Work out the finished part from the listing and answer in its coordinate system (mm). A direction names the side the tool comes from. Round coordinates to 2 decimals unless told otherwise and drop trailing zeros. Loops run counter-clockwise (first coordinate to the right, second up) from the corner with the lowest first, then second, coordinate; pieces in that order, holes last. Notation, with made-up numbers: (23.25, 66.5) -> (28.25, 66.5) arc R22 ccw to (28.25, 90.5) -> close; hole circle Ø2 at (-30, 17.25). An arc over 180 degrees is marked (long way). Write item = value, one per line. Start each with the question number.
```python
from build123d import *

# Parameters (mm, degrees)
F3_DEPTH = 12.13


with BuildPart() as f1:
    # F0 (on Front) → F1 (revolve)
    with BuildSketch(Plane.XZ):
        Polygon((20.5, 23.07), (20.5, 0), (23.37, 0), (23.37, 12.13), (21.62, 12.13), (21.62, 23.07), align=None)
    revolve(axis=Axis((0, 0, 6.4205313101), (0, 0, 1)))

    # F2 (on face) → F3 (join)
    with BuildSketch(Plane(origin=(0, 0, 0), x_dir=(1, 0, 0), z_dir=(0, 0, -1))):
        with BuildLine():
            ThreePointArc((-2.035, 23.2812301007), (0, 23.37), (2.035, 23.2812301007))
            ThreePointArc((2.035, 23.2812301007), (0, 25.37), (-2.035, 23.2812301007))
        make_face()
        with BuildLine():
            ThreePointArc((-7.9912848, 21.9612446652), (-6.048601084, 22.5736865604), (-4.059966687, 23.0146381788))
            ThreePointArc((-4.059966687, 23.0146381788), (-6.5662391743, 24.505538213), (-7.9912848, 21.9612446652))
        make_face()
        with BuildLine():
            ThreePointArc((-13.402976747, 19.1446366985), (-11.685, 20.2390136864), (-9.8782533536, 21.1796366985))
            ThreePointArc((-9.8782533536, 21.1796366985), (-12.685, 21.971064494), (-13.402976747, 19.1446366985))
        make_face()
        with BuildLine():
            ThreePointArc((-17.9012779783, 15.0233533788), (-16.5250854763, 16.5250854763), (-15.0233533788, 17.9012779783))
            ThreePointArc((-15.0233533788, 17.9012779783), (-17.9392990387, 17.9392990387), (-17.9012779783, 15.0233533788))
        make_face()
        with BuildLine():
            ThreePointArc((-21.1796366985, 9.8782533536), (-20.2390136864, 11.685), (-19.1446366985, 13.402976747))
            ThreePointArc((-19.1446366985, 13.402976747), (-21.971064494, 12.685), (-21.1796366985, 9.8782533536))
        make_face()
        with BuildLine():
            ThreePointArc((-23.0146381788, 4.059966687), (-22.5736865604, 6.048601084), (-21.9612446652, 7.9912848))
            ThreePointArc((-21.9612446652, 7.9912848), (-24.505538213, 6.5662391743), (-23.0146381788, 4.059966687))
        make_face()
        with BuildLine():
            ThreePointArc((-23.2812301007, -2.035), (-23.37, 0), (-23.2812301007, 2.035))
            ThreePointArc((-23.2812301007, 2.035), (-25.37, 0), (-23.2812301007, -2.035))
        make_face()
        with BuildLine():
            ThreePointArc((-23.0146381788, -4.059966687), (-24.505538213, -6.5662391743), (-21.9612446652, -7.9912848))
            ThreePointArc((-21.9612446652, -7.9912848), (-22.5736865604, -6.048601084), (-23.0146381788, -4.059966687))
        make_face()
        with BuildLine():
            ThreePointArc((-21.1796366985, -9.8782533536), (-21.971064494, -12.685), (-19.1446366985, -13.402976747))
            ThreePointArc((-19.1446366985, -13.402976747), (-20.2390136864, -11.685), (-21.1796366985, -9.8782533536))
        make_face()
        with BuildLine():
            ThreePointArc((-17.9012779783, -15.0233533788), (-17.9392990387, -17.9392990387), (-15.0233533788, -17.9012779783))
            ThreePointArc((-15.0233533788, -17.9012779783), (-16.5250854763, -16.5250854763), (-17.9012779783, -15.0233533788))
        make_face()
        with BuildLine():
            ThreePointArc((-13.402976747, -19.1446366985), (-12.685, -21.971064494), (-9.8782533536, -21.1796366985))
            ThreePointArc((-9.8782533536, -21.1796366985), (-11.685, -20.2390136864), (-13.402976747, -19.1446366985))
        make_face()
        with BuildLine():
            ThreePointArc((-7.9912848, -21.9612446652), (-6.5662391743, -24.505538213), (-4.059966687, -23.0146381788))
            ThreePointArc((-4.059966687, -23.0146381788), (-6.048601084, -22.5736865604), (-7.9912848, -21.9612446652))
        make_face()
        with BuildLine():
            ThreePointArc((-2.035, -23.2812301007), (0, -25.37), (2.035, -23.2812301007))
            ThreePointArc((2.035, -23.2812301007), (0, -23.37), (-2.035, -23.2812301007))
        make_face()
        with BuildLine():
            ThreePointArc((4.059966687, -23.0146381788), (6.5662391743, -24.505538213), (7.9912848, -21.9612446652))
            ThreePointArc((7.9912848, -21.9612446652), (6.048601084, -22.5736865604), (4.059966687, -23.0146381788))
        make_face()
        with BuildLine():
            ThreePointArc((9.8782533536, -21.1796366985), (12.685, -21.971064494), (13.402976747, -19.1446366985))
            ThreePointArc((13.402976747, -19.1446366985), (11.685, -20.2390136864), (9.8782533536, -21.1796366985))
        make_face()
        with BuildLine():
            ThreePointArc((15.0233533788, -17.9012779783), (17.9392990387, -17.9392990387), (17.9012779783, -15.0233533788))
            ThreePointArc((17.9012779783, -15.0233533788), (16.5250854763, -16.5250854763), (15.0233533788, -17.9012779783))
        make_face()
        with BuildLine():
            ThreePointArc((19.1446366985, -13.402976747), (21.971064494, -12.685), (21.1796366985, -9.8782533536))
            ThreePointArc((21.1796366985, -9.8782533536), (20.2390136864, -11.685), (19.1446366985, -13.402976747))
        make_face()
        with BuildLine():
            ThreePointArc((21.9612446652, -7.9912848), (24.505538213, -6.5662391743), (23.0146381788, -4.059966687))
            ThreePointArc((23.0146381788, -4.059966687), (22.5736865604, -6.048601084), (21.9612446652, -7.9912848))
        make_face()
        with BuildLine():
            ThreePointArc((23.2812301007, 2.035), (23.347796978, 1.0184676106), (23.37, 0))
            ThreePointArc((23.37, 0), (23.347796978, -1.0184676106), (23.2812301007, -2.035))
            ThreePointArc((23.2812301007, -2.035), (25.37, 0), (23.2812301007, 2.035))
        make_face()
        with BuildLine():
            ThreePointArc((21.9612446652, 7.9912848), (22.5736865604, 6.048601084), (23.0146381788, 4.059966687))
            ThreePointArc((23.0146381788, 4.059966687), (24.505538213, 6.5662391743), (21.9612446652, 7.9912848))
        make_face()
        with BuildLine():
            ThreePointArc((19.1446366985, 13.402976747), (20.2390136864, 11.685), (21.1796366985, 9.8782533536))
            ThreePointArc((21.1796366985, 9.8782533536), (21.971064494, 12.685), (19.1446366985, 13.402976747))
        make_face()
        with BuildLine():
            ThreePointArc((15.0233533788, 17.9012779783), (16.5250854763, 16.5250854763), (17.9012779783, 15.0233533788))
            ThreePointArc((17.9012779783, 15.0233533788), (17.9392990387, 17.9392990387), (15.0233533788, 17.9012779783))
        make_face()
        with BuildLine():
            ThreePointArc((9.8782533536, 21.1796366985), (11.685, 20.2390136864), (13.402976747, 19.1446366985))
            ThreePointArc((13.402976747, 19.1446366985), (12.685, 21.971064494), (9.8782533536, 21.1796366985))
        make_face()
        with BuildLine():
            ThreePointArc((4.059966687, 23.0146381788), (6.048601084, 22.5736865604), (7.9912848, 21.9612446652))
            ThreePointArc((7.9912848, 21.9612446652), (6.5662391743, 24.505538213), (4.059966687, 23.0146381788))
        make_face()
    extrude(amount=-F3_DEPTH)


solid = f1.part
```
Item 1: Section A-A (y = 0) is taken. Determine the outline of the cut face in (x, z).
Item 2: Flat-ended cylindrical pins translate along their axes: pin 1 (1 mm diameter, centred on y = -20, z = 16.5, fed in from +X); pin 2 (12 mm diameter, centred on x = -19, z = 14.5, fed in from +Y); pin 3 (1.5 mm diameter, centred on x = 3, z = 9, fed in from +Y). Find the tip coordinate at first contact, or state that the pin passes through.
Item 3: Find the intervals of material crossed by line 1 along X through (y, z) = (-18, 2.75); line 2 along Y through (x, z) = (0, 11); line 3 along Z through (x, y) = (-14, 18), in increasing order. Write a range as [from, to].
Item 4: A tool of negligible diameter and unlimited length cuts with its end or side. For faces 5 (the cylindrical face through (18.53, -14.24, 6.15)), 6 (the flat face through (0, 21, 0)), 7 (the cylindrical face through (23.17, -3.06, 6.15)), from which of +Z, -Z, +X, -X, +Y, -Y can it reach the whole face along a straight path? Write none if from no direction.
Item 5: Section C-C (z = 21.5) is taken. Determine the outline of the cut face in (x, y), then the cut area to 3 significant figures.
Item 6: The mould has two halves that part along Y. Classify faces 1 (the cylindrical face through (-3.04, 23.17, 6.15)), 2 (the cylindrical face through (3.04, -23.17, 6.15)), 3 (the cylindrical face through (17.97, -17.91, 5.98)), 4 (the flat face through (11, 19, 12.13)): pulls with the +Y half, pulls with the -Y half, needs draft (parallel to the pull), parting line crosses it, or undercut.
Worked answers:
q1.outline = (-25.37, 0) -> (-20.5, 0) -> (-20.5, 23.07) -> (-21.62, 23.07) -> (-21.62, 12.13) -> (-25.37, 12.13) -> close; (20.5, 0) -> (25.37, 0) -> (25.37, 12.13) -> (21.62, 12.13) -> (21.62, 23.07) -> (20.5, 23.07) -> close
q2.pin_1 = 9.34
q2.pin_2 = 21.12
q2.pin_3 = 23.26
q3.line_1 = [-17.88, -15.12], [-14.9, -9.81], [9.81, 14.9], [15.12, 17.88]
q3.line_2 = [-25.37, -20.5], [20.5, 25.37]
q3.line_3 = [0, 12.13]
q4.face_5 = +Z, -Z
q4.face_6 = -Z, +X, -X, +Y, -Y
q4.face_7 = +Z, -Z, +X
q5.outline = circle Ø43.24 at (0, 0); hole circle Ø41 at (0, 0)
q5.area = 148 mm2
q6.face_1 = pulls with the +Y half
q6.face_2 = pulls with the -Y half
q6.face_3 = undercut
q6.face_4 = needs draft
